Geometry: final body of the model. Coordinates: model frame, mm. Face numbers are marked on the shaded views. A direction names the side the tool comes from. Give positions to 0.01 mm unless a question says otherwise; leave off trailing zeros. Loops run counter-clockwise (first coordinate to the right, second up) from the corner with the lowest first, then second, coordinate; pieces in that order, holes last. Notation, with made-up numbers: M 17.25,87 L 45.25,87 A25 cw 45.25,111 Z; hole C 82.25,-29.5 d10. An arc over 180 degrees is marked long. One line per question, with ' | ' between items. Start each with the question number.
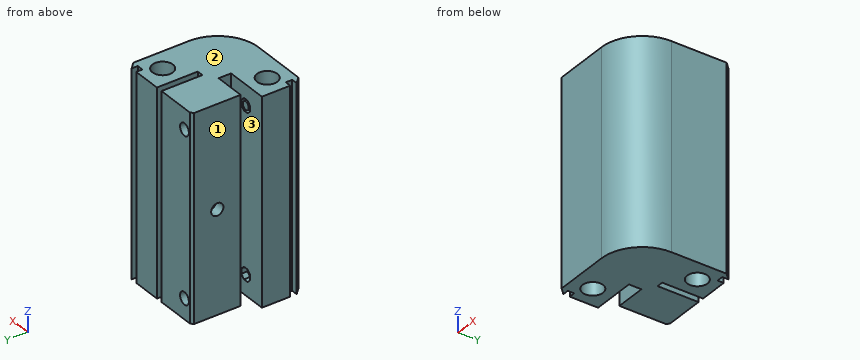
Solid Edge part; units mm, degrees
sketch "Sketch1" plane through (0, 0, 0) normal (0, 0, -1) x (-1, 0, 0)
  line L0 (-200, -100) -> (200, -100)
  line L1 (200, -100) -> (200, 100)
  line L2 (200, 100) -> (-200, 100)
  line L3 (-200, 100) -> (-200, -100)
extrude "Protrusion1" add sketch "Sketch1" against normal blind 250
sketch "Sketch2" plane through (0, 0, 0) normal (0, 0, -1) x (-1, 0, 0)
  circle A0 centre (100, 0) radius 50
  dimension "D1" = 200
extrude "Cutout1" cut sketch "Sketch2" against normal blind 3
fillet "Round_8" radius 20 4 edges at (200, -100, 125) (200, 100, 125) (-200, 100, 125) (-200, -100, 125)
fillet "Round_9" radius 30 8 edges at (0, -100, 0) (-194.1421, -94.1421, 0) (-200, 0, 0) (-194.1421, 94.1421, 0) (0, 100, 0) (194.1421, 94.1421, 0) (200, 0, 0) (194.1421, -94.1421, 0)
sketch "Sketch3" plane through (200, 0, 140) normal (1, 0, 0) x (0, -1, 0)
  line L0 (70, 57.1371) -> (-70, 57.1371)
  line L1 (-70, 57.1371) -> (-70, 97.1371)
  line L2 (-70, 97.1371) -> (70, 97.1371)
  line L3 (70, 97.1371) -> (70, 57.1371)
  dimension "D1" = 70
extrude "ExtrudedCutout_37" cut sketch "Sketch3" against normal blind 30
sketch "Sketch4" plane through (185, 0, 82.8629) normal (0, 0, -1) x (0, -1, 0)
  line L0 (-70, 15) -> (70, 15)
  line L1 (70, 15) -> (70, 10)
  line L2 (70, 10) -> (-70, 10)
  line L3 (-70, 10) -> (-70, 15)
extrude "Cutout2" cut sketch "Sketch4" against normal blind 5
sketch "Sketch5" plane through (185, 0, 42.8629) normal (0, 0, 1) x (0, -1, 0)
  line L0 (-70, -10) -> (70, -10)
  line L1 (70, -10) -> (70, -15)
  line L2 (70, -15) -> (-70, -15)
  line L3 (-70, -15) -> (-70, -10)
extrude "ExtrudedCutout_39" cut sketch "Sketch5" against normal blind 5
sketch "Sketch6" plane through (185, 70, 62.8629) normal (0, -1, 0) x (1, 0, 0)
  line L0 (-15, 25) -> (-10, 25)
  line L1 (-10, 25) -> (-10, -25)
  line L2 (-10, -25) -> (-15, -25)
  line L3 (-15, -25) -> (-15, 25)
extrude "Cutout3" cut sketch "Sketch6" against normal blind 5
sketch "Sketch7" plane through (185, -70, 62.8629) normal (0, 1, 0) x (1, 0, 0)
  line L0 (-15, 25) -> (-10, 25)
  line L1 (-10, 25) -> (-10, -25)
  line L2 (-10, -25) -> (-15, -25)
  line L3 (-15, -25) -> (-15, 25)
extrude "Cutout4" cut sketch "Sketch7" against normal blind 5
sketch "Sketch8" plane through (170, 0, 62.8629) normal (1, 0, 0) x (0, -1, 0)
  line L0 (-75, 25) -> (75, 25)
  line L1 (75, 25) -> (75, -25)
  line L2 (75, -25) -> (-75, -25)
  line L3 (-75, -25) -> (-75, 25)
  line L4 (72, 22.1284) -> (-72, 22.1284)
  line L5 (-72, 22.1284) -> (-72, -21.8716)
  line L6 (-72, -21.8716) -> (72, -21.8716)
  line L7 (72, -21.8716) -> (72, 22.1284)
  dimension "D1" = 75
extrude "ExtrudedCutout_42" cut sketch "Sketch8" along normal mid plane 10
sketch "Sketch9" plane through (200, 0, 140) normal (1, 0, 0) x (0, -1, 0)
  circle A0 centre (0, -30) radius 68.3204
extrude "Cutout5" cut sketch "Sketch9" against normal blind 6
sketch "Sketch10" plane through (0, 0, 250) normal (0, 0, 1) x (-1, 0, 0)
  line L0 (-180, 100) -> (180, 100)
  line L1 (180, 100) -> (180, 97)
  line L2 (180, 97) -> (-180, 97)
  line L3 (-180, 97) -> (-180, 100)
  line L4 (200, 80) -> (197, 80)
  line L5 (197, 80) -> (197, -80)
  line L6 (197, -80) -> (200, -80)
  line L7 (200, -80) -> (200, 80)
  line L8 (-200, 80) -> (-197, 80)
  line L9 (-197, 80) -> (-197, -80)
  line L10 (-197, -80) -> (-200, -80)
  line L11 (-200, -80) -> (-200, 80)
  line L12 (-180, -100) -> (180, -100)
  line L13 (180, -100) -> (180, -97)
  line L14 (180, -97) -> (-180, -97)
  line L15 (-180, -97) -> (-180, -100)
extrude "Cutout6" cut sketch "Sketch10" against normal blind 220
sketch "Sketch11" plane through (165, -97, 140) normal (0, -1, 0) x (0, 0, 1)
  line L0 (-110, 23.978) -> (116.0147, 23.978)
  line L1 (116.0147, 23.978) -> (116.0147, -38.9945)
  line L2 (116.0147, -38.9945) -> (-110, -38.9945)
  line L3 (-110, -38.9945) -> (-110, 23.978)
extrude "ExtrudedCutout_47" cut sketch "Sketch11" along normal mid plane 474
sketch "Sketch12" plane through (0, 0, 0) normal (0, 0, -1) x (-1, 0, 0)
  line L0 (-150, -121.4584) -> (-150, -50)
  line L1 (-254.1695, -50) -> (-150, -50)
  line L2 (-254.1695, -50) -> (-254.1695, 113.1592)
  line L3 (-254.1695, 113.1592) -> (264.7141, 113.1592)
  line L4 (264.7141, 113.1592) -> (271.856, -149.5027)
  line L5 (271.856, -149.5027) -> (-150, -121.4584)
extrude "ExtrudedCutout_46" cut sketch "Sketch12" against normal blind 317
sketch "Sketch13" plane through (175, -75, 30) normal (0, 0, 1) x (0, 1, 0)
  line L0 (17.7429, 25) -> (30.7571, 11.9857)
  line L1 (29.3143, 29.7) -> (30.7571, 11.9857)
  line L2 (17.7429, 25) -> (29.3143, 29.7)
extrude "Cutout7" cut sketch "Sketch13" against normal blind 15
sketch "Sketch14" plane through (153.6286, -53.6286, 22.5) normal (-0.7071, 0.7071, 0) x (0.7071, 0.7071, 0)
  line L0 (-5.1316, -2.5) -> (5.1316, -2.5)
  line L1 (5.1316, 2.97) -> (5.1316, -2.5)
  line L2 (-5.1316, 2.97) -> (5.1316, 2.97)
  line L3 (-5.1316, 2.97) -> (-5.1316, -2.5)
  dimension "D1" = 5.1316
extrude "ExtrudedCutout_49" cut sketch "Sketch14" against normal blind 46
sketch "Sketch15" plane through (175, -75, 30) normal (0, 0, 1) x (0, -1, 0)
  circle A0 centre (-17.7429, -17.7429) radius 1.5
extrude "ExtrudedCutout_50" cut sketch "Sketch15" against normal blind 9
sketch "Sketch16" plane through (175, -75, 30) normal (0, 0, 1) x (0, -1, 0)
  line L0 (5, -20) -> (-3, -20)
  line L1 (-3, -20) -> (-3, -15)
  line L2 (5, -15) -> (-3, -15)
  line L3 (5, -20) -> (5, -15)
  line L4 (-20, 5) -> (-20, -3)
  line L5 (-20, -3) -> (-15, -3)
  line L6 (-15, 5) -> (-15, -3)
  line L7 (-20, 5) -> (-15, 5)
  dimension "D1" = 5
  dimension "D2" = 3
extrude "Cutout8" cut sketch "Sketch16" against normal blind 10
sketch "Sketch17" plane through (175, -50, 15) normal (0, 1, 0) x (0, 0, 1)
  circle A0 centre (10, 1) radius 1.5
extrude "Cutout9" cut sketch "Sketch17" against normal blind 8
sketch "Sketch18" plane through (150, -75, 15) normal (-1, 0, 0) x (0, -1, 0)
  circle A0 centre (1.0029, 10) radius 1.5
extrude "Cutout10" cut sketch "Sketch18" against normal blind 9
sketch "Sketch19" plane through (150, -75, 15) normal (-1, 0, 0) x (0, -1, 0)
  circle A0 centre (-17, -7) radius 5
  circle A1 centre (14.7841, 4.53) radius 5
extrude "Cutout11" cut sketch "Sketch19" against normal blind 2
sketch "Sketch20" plane through (175, -50, 15) normal (0, 1, 0) x (-1, 0, 0)
  circle A0 centre (17, -7) radius 5
  circle A1 centre (-14.7841, 4.53) radius 5
extrude "Cutout12" cut sketch "Sketch20" against normal blind 2
fillet "Round_16" radius 5 1 edges at (153.6286, -53.6286, 15)
sketch "Sketch21" plane through (175, -75, 30) normal (0, 0, 1) x (0, -1, 0)
  circle A0 centre (-15, 14.7841) radius 5
  circle A1 centre (14.7841, -15) radius 5
extrude "ExtrudedCutout_56" cut sketch "Sketch21" against normal blind 3
sketch "Sketch22" plane through (169.892, -69.892, 19.53) normal (0, 0, 1) x (0.7071, -0.7071, 0)
  line L0 (23, 5.1316) -> (-12.8442, 5.1316)
  line L1 (-12.8442, 5.1316) -> (-12.8442, -5.1316)
  line L2 (-12.8442, -5.1316) -> (23, -5.1316)
  line L3 (23, -5.1316) -> (23, 5.1316)
extrude "ExtrudedProtrusion_20" add sketch "Sketch22" along normal blind 6
sketch "Sketch23" plane through (175, -75, 30) normal (0, 0, 1) x (0, -1, 0)
  arc A0 (5, 25) -> (25, 5) centre (5, 5) cw
  line L0 (25, 5) -> (25, -25)
  line L1 (25, -25) -> (-17.7429, -25)
  line L2 (-17.7429, -25) -> (-25, -17.7429)
  line L3 (-25, -17.7429) -> (-25, 25)
  line L4 (-25, 25) -> (5, 25)
  circle A1 centre (-15, 14.7841) radius 5
  circle A2 centre (14.7841, -15) radius 5
extrude "Protrusion2" add sketch "Sketch23" along normal blind 100
sketch "Sketch24" plane through (153.6286, -53.6286, 77.5) normal (-0.7071, 0.7071, 0) x (0, 0, 1)
  line L0 (-47.5, -40.0408) -> (-85.2138, -40.0408)
  line L1 (-85.2138, -40.0408) -> (-85.2138, 45.7641)
  line L2 (-85.2138, 45.7641) -> (-47.5, 45.7641)
  line L3 (-47.5, 45.7641) -> (-47.5, -40.0408)
extrude "ExtrudedCutout_57" cut sketch "Sketch24" along normal mid plane 148
sketch "Sketch25" plane through (175, -75, 130) normal (0, 0, 1) x (0, -1, 0)
  line L0 (-22, 22) -> (-22, 18.85)
  line L1 (-22, 18.85) -> (-25, 18.85)
  line L2 (-29.2429, 28.0796) -> (-25, 18.85)
  line L3 (-22, 28.0796) -> (-29.2429, 28.0796)
  line L4 (-22, 25) -> (-22, 28.0796)
  line L5 (-25, 22) -> (-22, 25)
  line L6 (-22, 22) -> (-25, 22)
  line L7 (22, -22) -> (18.85, -22)
  line L8 (18.85, -22) -> (18.85, -25)
  line L9 (28.0796, -29.2429) -> (18.85, -25)
  line L10 (28.0796, -22) -> (28.0796, -29.2429)
  line L11 (25, -22) -> (28.0796, -22)
  line L12 (22, -25) -> (25, -22)
  line L13 (22, -22) -> (22, -25)
extrude "Cutout13" cut sketch "Sketch25" against normal blind 148
sketch "Sketch26" plane through (175, -75, 130) normal (0, 0, 1) x (0, -1, 0)
  line L0 (5, -4) -> (5, -25)
  line L1 (5, -25) -> (-1.1, -25)
  line L2 (-1.1, -25) -> (-1.1, -4)
  line L3 (5, -4) -> (-1.1, -4)
extrude "ExtrudedCutout_60" cut sketch "Sketch26" against normal blind 186
sketch "Sketch27" plane through (160, -80, 80) normal (0, 1, 0) x (0, 0, 1)
  line L0 (-38.7574, -1.9959) -> (-41.2426, -1.9959)
  line L1 (-41.2426, -1.9959) -> (-43, -0.2385)
  line L2 (-43, -0.2385) -> (-43, 2.2467)
  line L3 (-43, 2.2467) -> (-41.2426, 4.0041)
  line L4 (-41.2426, 4.0041) -> (-38.7574, 4.0041)
  line L5 (-38.7574, 4.0041) -> (-37, 2.2467)
  line L6 (-37, 2.2467) -> (-37, -0.2385)
  line L7 (-37, -0.2385) -> (-38.7574, -1.9959)
  line L8 (38.7574, -1.9959) -> (41.2426, -1.9959)
  line L9 (41.2426, -1.9959) -> (43, -0.2385)
  line L10 (43, -0.2385) -> (43, 2.2467)
  line L11 (43, 2.2467) -> (41.2426, 4.0041)
  line L12 (41.2426, 4.0041) -> (38.7574, 4.0041)
  line L13 (38.7574, 4.0041) -> (37, 2.2467)
  line L14 (37, 2.2467) -> (37, -0.2385)
  line L15 (37, -0.2385) -> (38.7574, -1.9959)
  circle A0 centre (40, 1.0041) radius 2
extrude "Cutout14" cut sketch "Sketch27" against normal blind 3
sketch "Sketch28" plane through (160, -80, 80) normal (0, 1, 0) x (0, 0, 1)
  circle A0 centre (-40, 1.0041) radius 2
  circle A1 centre (40, 1.0041) radius 2
extrude "ExtrudedCutout_62" cut sketch "Sketch28" along normal blind 43
sketch "Sketch29" plane through (177.0686, -50, 80) normal (0, 1, 0) x (-1, 0, 0)
  circle A0 centre (16.0645, 40) radius 3
  circle A1 centre (16.0645, -40) radius 3
extrude "Cutout15" cut sketch "Sketch29" against normal blind 5
sketch "Sketch30" plane through (175, -75, 130) normal (0, 0, 1) x (0, -1, 0)
  line L0 (-1.1, -18.9657) -> (-27.9226, -18.9657)
  line L1 (-27.9226, -18.9657) -> (-17.7429, -25)
  line L2 (-17.7429, -25) -> (-1.1, -25)
  line L3 (-1.1, -25) -> (-1.1, -18.9657)
extrude "Cutout16" cut sketch "Sketch30" against normal blind 148
sketch "Sketch31" plane through (175, -75, 30) normal (0, 0, -1) x (0, 1, 0)
  line L0 (25, 4.7841) -> (5, 4.7841)
  line L1 (5, 4.7841) -> (5, 1.6341)
  line L2 (5, 1.6341) -> (25, 1.6341)
  line L3 (25, 1.6341) -> (25, 4.7841)
extrude "Cutout17" cut sketch "Sketch31" against normal blind 246
sketch "Sketch32" plane through (156.0343, -62.5614, 80) normal (-1, 0, 0) x (0, -1, 0)
  circle A0 centre (-0.0614, 0) radius 2
extrude "Cutout18" cut sketch "Sketch32" against normal blind 30
sketch "Sketch33" plane through (156.0343, -62.5614, 80) normal (-1, 0, 0) x (0, -1, 0)
  circle A0 centre (-0.0614, 0) radius 3
extrude "Cutout19" cut sketch "Sketch33" against normal blind 5
sketch "Sketch34" plane through (179.7841, -60, 80) normal (-1, 0, 0) x (0, 0, 1)
  line L0 (3, -3.7426) -> (3, -1.2574)
  line L1 (3, -1.2574) -> (1.2426, 0.5)
  line L2 (1.2426, 0.5) -> (-1.2426, 0.5)
  line L3 (-1.2426, 0.5) -> (-3, -1.2574)
  line L4 (-3, -1.2574) -> (-3, -3.7426)
  line L5 (-3, -3.7426) -> (-1.2426, -5.5)
  line L6 (-1.2426, -5.5) -> (1.2426, -5.5)
  line L7 (1.2426, -5.5) -> (3, -3.7426)
extrude "Cutout20" cut sketch "Sketch34" against normal blind 3
Q1. Section A-A, the plane y = -67.5. Output: boundary loops of the cut face in (x, z).
Q2. Set-up query: the marked faces 1, 2 and 3. Return all of +Z, -Z, +X, -X, +Y, -Y with unobstructed straight access to the full face (end or side cutting, diameter ignored); none if empty.
Q3. Section B-B, the plane y = -92. Output: boundary loops of the cut face in (x, z).
Q4. Material intervals for L1, parallel to Y at x = 159.5, z = 58.5; L2, parallel to X at y = -60, z = 88.5; L3, parallel to Z at x = 160, y = -73.5, sorted ascending.
Q5. Section D-D, the plane y = -86. Output: boundary loops of the cut face in (x, z), plus the area to 3 significant figures.
Q6. Section C-C, the plane z = 72.5. Output: boundary loops of the cut face in (x, y), plus the area to 3 significant figures.
Q7. Contact query for flat-ended pins moving along their axis: pin 1 (1.2 mm diameter, centred on y = -82, z = 40, fed in from +X); pin 2 (0.6 mm diameter, centred on y = -64, z = 80.5, fed in from -X); pin 3 (3.5 mm diameter, centred on x = 161, z = 40, fed in from +Y); pin 4 (10 mm diameter, centred on x = 158.5, y = -74, fed in from +Z). Output: stop coordinate, or through.
Model answer:
1) outline: M 156.03,30 L 176.63,30 L 176.63,130 L 156.03,130 Z; M 179.78,30 L 200,30 L 200,130 L 179.78,130 Z; hole C 161,40 d4; hole C 161,120 d4
2) face 1: +Z, -Z, -X, +Y | face 2: +Z, +X, -X, +Y, -Y | face 3: +Z, -Z, -X
3) outline: M 150,30 L 155.52,30 L 155.52,130 L 150,130 Z; M 164.48,30 L 196,30 L 196,130 L 164.48,130 Z
4) L1: y = -100 to -94.76, -84.81 to -80, -73.9 to -50 | L2: x = 156.03 to 176.63, 179.78 to 184.78, 194.78 to 200 | L3: z = 30 to 38.27, 41.73 to 118.27, 121.73 to 130
5) outline: M 150,30 L 156.73,30 L 156.73,130 L 150,130 Z; M 163.27,30 L 199.08,30 L 199.08,130 L 163.27,130 Z | area: 4,250 mm^2
6) outline: M 150,-97 L 153,-100 L 180,-100 A20 ccw 200,-80 L 200,-53 L 197,-50 L 197,-53 L 193.85,-53 L 193.85,-50 L 179.78,-50 L 179.78,-70 L 176.63,-70 L 176.63,-50 L 157.26,-50 L 156.03,-51.22 L 156.03,-73.9 L 171,-73.9 L 171,-80 L 150,-80 L 150,-93.85 L 153,-93.85 L 153,-97 Z; hole C 160,-89.78 d10; hole C 189.78,-60 d10 | area: 1,890 mm^2
7) pin 1: stops at x = 199.95 | pin 2: stops at x = 186.03 | pin 3: stops at y = -83 | pin 4: stops at z = 130
